Check sheet for the modelled part. Datum: model origin and axes. Units: mm. A direction names the side the tool comes from. Coordinates: 2 decimals unless noted, no trailing zeros. Order: outer loops, then holes, each group sorted by start corner. A loop starts at its lowest first (then second) coordinate and runs counter-clockwise, first axis right, second up.
from build123d import *

# Parameters (mm, degrees)
BOSS_EXTRUDE1_DEPTH = 5
SKETCH3_R           = 9.95
BOSS_EXTRUDE2_DEPTH = 2
SKETCH4_R           = 1.5
CUT_EXTRUDE1_DEPTH  = 64.639610307
SKETCH5_R           = 1.4
CUT_EXTRUDE2_DEPTH  = 63.649820431
FILLET1_R           = 2
FILLET2_R           = 0.5


with BuildPart() as part:
    # Sketch1 → Revolve1 (revolve)
    with BuildSketch(Plane(origin=(0, 0, 0), x_dir=(1, 0, 0), z_dir=(0, 1, 0))):
        Polygon((0, 0), (9.95, 0), (9.95, 7), (11.5, 7), (12.5, 8), (0, 8), align=None)
    revolve(axis=Axis((0, 0, 0), (0, 0, -1)))

    # Sketch2 → Boss-Extrude1 (add)
    with BuildSketch(Plane(origin=(0, 0, -8), x_dir=(-1, 0, 0), z_dir=(0, 0, -1))):
        with BuildLine():
            Line((0, 15), (60, 15))
            Line((60, 15), (60, -15))
            Line((60, -15), (0, -15))
            ThreePointArc((0, -15), (-15, 0), (0, 15))
        make_face()
    extrude(amount=BOSS_EXTRUDE1_DEPTH)

    # Sketch3 → Boss-Extrude2 (add)
    with BuildSketch(Plane.XY):
        Circle(SKETCH3_R)
    extrude(amount=BOSS_EXTRUDE2_DEPTH)

    # Sketch4 → Cut-Extrude1 (cut, through all)
    with BuildSketch(Plane.XY.offset(2)):
        with Locations((0, 7)):
            Circle(SKETCH4_R)
        with Locations((7, 0)):
            Circle(SKETCH4_R)
        with Locations((0, -7)):
            Circle(SKETCH4_R)
        with Locations((-7, 0)):
            Circle(SKETCH4_R)
    extrude(amount=-CUT_EXTRUDE1_DEPTH, mode=Mode.SUBTRACT)

    # Sketch5 → Cut-Extrude2 (cut, through all)
    with BuildSketch(Plane.XY.offset(-8)):
        with Locations((-55, 10)):
            Circle(SKETCH5_R)
        with Locations((-55, -10)):
            Circle(SKETCH5_R)
        with Locations((-40, 10)):
            Circle(SKETCH5_R)
        with Locations((-40, -10)):
            Circle(SKETCH5_R)
        with Locations((-25, 10)):
            Circle(SKETCH5_R)
        with Locations((-25, -10)):
            Circle(SKETCH5_R)
    extrude(amount=-CUT_EXTRUDE2_DEPTH, mode=Mode.SUBTRACT)

    # Fillet1
    fillet1_edges = [part.edges().sort_by_distance(p)[0] for p in [
        (-60, -15, -10.5),
        (-60, 15, -10.5),
    ]]
    fillet(fillet1_edges, radius=FILLET1_R)

    # Fillet2
    fillet2_edges = [part.edges().sort_by_distance(p)[0] for p in [
        (-9.95, 0, 2),
    ]]
    fillet(fillet2_edges, radius=FILLET2_R)


solid = part.part
(1) Cross-section at C-C (x = -36.5). Enter the section's corners in (y, z).
Filled in:
outline: (-15, -13) - (15, -13) - (15, -8) - (-15, -8) - close
(2) Go/stop test with flat-tipped pins: P1, Ø3.5, axis at x = -55, y = 10, coming from the +Z side; P2, Ø1.8, axis at x = 7, y = 0, coming from the -Z side; P3, Ø1.5, axis at x = 6.5, z = -3, coming from the -Y side; P4, Ø8, axis at y = -9, z = -11.5, coming from the +X side. Record where each tip stops, or that it passes through.
Filled in:
P1: stops at z = -8
P2: passes through
P3: stops at y = -8.12
P4: stops at x = 14.14
(3) Cross-section at B-B (z = -3). Enter the section's corners in (x, y), and give its area (3 significant figures).
Filled in:
outline: circle Ø19.9 at (0, 0); hole circle Ø3 at (-7, 0); hole circle Ø3 at (0, -7); hole circle Ø3 at (0, 7); hole circle Ø3 at (7, 0)
area: 283 mm2
(4) Tool access check on faces 5 (the cylindrical face through (-7.9, -6.05, -2.81)), 6 (the cylindrical face through (15, 0, -10)). Record the directions out of +Z, -Z, +X, -X, +Y, -Y that give a thin tool (end or side, any length) a straight path to the whole face; none if there is none.
Filled in:
face 5: +Z
face 6: +Z, -Z, +X
(5) Release check for a two-part mould opening along Y. For faces 1 (the flat face through (-29, -15, -10)), 2 (the flat face through (-60, 0, -10)), 3 (the cylindrical face through (-0.325, -8.464, -5.395)), 4 (the cylindrical face through (-23.71, -10.54, -10.46)) record: +Y half, -Y half, draft (parallel to the pull), parting line (faces both ways), or undercut.
Filled in:
face 1: -Y half
face 2: draft
face 3: undercut
face 4: undercut
(6) Thickness scan on probe 1 along Y at (x, z) = (-25, -10.2); probe 2 along X at (y, z) = (0.25, 0.5); probe 3 along Y at (x, z) = (-0.5, -12). Record the ranges inside material, lowest first.
Filled in:
probe 1: y = -15 to -11.4, -8.6 to 8.6, 11.4 to 15
probe 2: x = -9.95 to -8.48, -5.52 to 5.52, 8.48 to 9.95
probe 3: y = -15 to -8.41, -5.59 to 5.59, 8.41 to 15
(7) Cross-section at A-A (z = -11.5). Count the separate pieces of the cut face and the enclosed holes in it, and give its area (3 significant figures).
Filled in:
separate pieces: 1
enclosed holes: 10
area: 2,090 mm2
